from build123d import *

# Parameters (mm, degrees)
SKETCH1_R           = 5.1
SKETCH1_R_2         = 2.2
BOSS_EXTRUDE1_DEPTH = 7
SKETCH1_3_R         = 5.1
SKETCH1_3_R_2       = 2.2
CUT_EXTRUDE1_DEPTH  = 5.5
SKETCH1_4_R         = 2.2
CUT_EXTRUDE2_DEPTH  = 7


with BuildPart() as part:
    # Sketch1 → Boss-Extrude1 (new body)
    with BuildSketch(Plane.XY):
        Polygon((54.5, 26.172980381), (54.5, 62.5), (5.5, 62.5), (5.5, 26.172980381), (-8.376844495, 18.161180477), (0, 0), (60, 0), (68.376844495, 18.161180477), align=None)
        with Locations((29.999295859, 51.499999991)):
            Circle(SKETCH1_R, mode=Mode.SUBTRACT)
        with Locations((5.800227015, 13.687854711)):
            Circle(SKETCH1_R, mode=Mode.SUBTRACT)
        with Locations((54.200362799, 13.689133529)):
            Circle(SKETCH1_R, mode=Mode.SUBTRACT)
        with Locations((5.800227015, 13.687854711)):
            Circle(SKETCH1_R)
        with Locations((5.800227015, 13.687854711)):
            Circle(SKETCH1_R_2, mode=Mode.SUBTRACT)
        with Locations((5.800227015, 13.687854711)):
            Circle(SKETCH1_R_2)
        with Locations((54.200362799, 13.689133529)):
            Circle(SKETCH1_R)
        with Locations((54.200362799, 13.689133529)):
            Circle(SKETCH1_R_2, mode=Mode.SUBTRACT)
        with Locations((54.200362799, 13.689133529)):
            Circle(SKETCH1_R_2)
        with Locations((29.999295859, 51.499999991)):
            Circle(SKETCH1_R)
        with Locations((29.999295859, 51.499999991)):
            Circle(SKETCH1_R_2, mode=Mode.SUBTRACT)
        with Locations((29.999295859, 51.499999991)):
            Circle(SKETCH1_R_2)
    extrude(amount=BOSS_EXTRUDE1_DEPTH)

    # Sketch1<3> → Cut-Extrude1 (cut)
    with BuildSketch(Plane.XY):
        with Locations((29.999295859, 51.499999991)):
            Circle(SKETCH1_3_R)
        with Locations((29.999295859, 51.499999991)):
            Circle(SKETCH1_3_R_2, mode=Mode.SUBTRACT)
        with Locations((54.200362799, 13.689133529)):
            Circle(SKETCH1_3_R)
        with Locations((54.200362799, 13.689133529)):
            Circle(SKETCH1_3_R_2, mode=Mode.SUBTRACT)
        with Locations((5.800227015, 13.687854711)):
            Circle(SKETCH1_3_R)
        with Locations((5.800227015, 13.687854711)):
            Circle(SKETCH1_3_R_2, mode=Mode.SUBTRACT)
    extrude(amount=CUT_EXTRUDE1_DEPTH, mode=Mode.SUBTRACT)

    # Sketch1<4> → Cut-Extrude2 (cut)
    with BuildSketch(Plane.XY):
        with Locations((54.200362799, 13.689133529)):
            Circle(SKETCH1_4_R)
        with Locations((5.800227015, 13.687854711)):
            Circle(SKETCH1_4_R)
        with Locations((29.999295859, 51.499999991)):
            Circle(SKETCH1_4_R)
    extrude(amount=CUT_EXTRUDE2_DEPTH, mode=Mode.SUBTRACT)


solid = part.part
For this review, take the finished solid that the model builds, in its own axes (mm). A direction names the side the tool comes from. Coordinates: 2 decimals unless noted, no trailing zeros. Order: outer loops, then holes, each group sorted by start corner. A loop starts at its lowest first (then second) coordinate and runs counter-clockwise, first axis right, second up. Notation, with made-up numbers: (-15.75, -10.5) - (6.25, -10.5) arc R15 ccw to (6.25, -4.5) - close; hole circle Ø10 at (50.5, 48). An arc over 180 degrees is marked (long way). Use one line per item in the form item = value.
Q1. For P1, Ø3.5, axis at y = 37, z = 2, coming from the -X side; P2, Ø3, axis at x = 57, z = 3.5, coming from the +Y side; P3, Ø8, axis at x = 5.8, y = 13.69, coming from the -Z side; P4, Ø4, axis at x = 54.2, y = 13.69, coming from the +Z side, all flat-tipped, find the tip position at first contact; note any pin that passes through.
Checked values:
P1 = 5.5
P2 = 25.6
P3 = 5.5
P4 = through
Q2. Consider section B-B (z = 1.25). Give the boundary of the cut face in (x, y), then the cut area to 3 significant figures.
Checked values:
outline = (-8.38, 18.16) - (0, 0) - (60, 0) - (68.38, 18.16) - (54.5, 26.17) - (54.5, 62.5) - (5.5, 62.5) - (5.5, 26.17) - close; hole circle Ø10.2 at (5.8, 13.69); hole circle Ø10.2 at (30, 51.5); hole circle Ø10.2 at (54.2, 13.69)
area = 3,280 mm2
Q3. Draft analysis for pull direction Y (two halves, no side actions). For faces 4 (the flat face through (54.5, 44, 3)), 5 (the cylindrical face through (58.911, 11.736, 2.712)), 6 (the flat face through (-1.341, 22.223, 3.451)), state which applies: +Y half, -Y half, draft (parallel to the pull), parting line (faces both ways), or undercut.
Checked values:
face_4 = draft
face_5 = undercut
face_6 = +Y half
Q4. For probe 1 along X at (y, z) = (18, 2.75); probe 2 along X at (y, z) = (29, 2.25); probe 3 along Y at (x, z) = (33, 0.5), list the stretches that pass through material, from the lowest coordinate up. Write a range as from..to.
Checked values:
probe_1 = -8.3..3.08, 8.52..51.48, 56.93..68.3
probe_2 = 5.5..54.5
probe_3 = 0..47.38, 55.62..62.5
Q5. Consider section C-C (x = 9.5). Give the boundary of the cut face in (y, z).
Checked values:
outline = (0, 0) - (10.18, 0) - (10.18, 5.5) - (17.2, 5.5) - (17.2, 0) - (62.5, 0) - (62.5, 7) - (0, 7) - close
Q6. Consider section D-D (y = 34). Give the boundary of the cut face in (x, z), then the cut area to 3 significant figures.
Checked values:
outline = (5.5, 0) - (54.5, 0) - (54.5, 7) - (5.5, 7) - close
area = 343 mm2
Q7. For faces 1 (the cylindrical face through (28.894, 46.521, 2.712)), 2 (the flat face through (30, 0, 3)), 3 (the flat face through (5.5, 45, 3)), list the 3-axis set-ups (+Z, -Z, +X, -X, +Y, -Y) from which the entire face can be reached by the end or side of a thin tool; tool diameter is ignored.
Checked values:
face_1 = -Z
face_2 = +Z, -Z, +X, -X, -Y
face_3 = +Z, -Z, -X, +Y
Q8. Consider section A-A (y = 51.5). Give the boundary of the cut face in (x, z), then the cut area to 3 significant figures.
Checked values:
outline = (5.5, 0) - (24.9, 0) - (24.9, 5.5) - (27.8, 5.5) - (27.8, 7) - (5.5, 7) - close; (32.2, 5.5) - (35.1, 5.5) - (35.1, 0) - (54.5, 0) - (54.5, 7) - (32.2, 7) - close
area = 280 mm2
